The drawing under review shows one solid part. Ordinate dimensions are in mm from its lowest x, y, z. A direction names the side the tool comes from. Round coordinates to 2 decimals unless told otherwise and drop trailing zeros. Order: outer loops, then holes, each group sorted by start corner. A loop starts at its lowest first (then second) coordinate and runs counter-clockwise, first axis right, second up.
1) Consider section C-C (z = 79). Give the boundary of the cut face in (x, y).
2) Machinability: for the marked faces 1 and 2, which of the approach directions +Z, -Z, +X, -X, +Y, -Y give a long, thin tool a straight path to every point of the face, cutting with its end or side? Answer none if there is none.
3) Consider section A-A (y = 32). Give the boundary of the cut face in (x, z), then the cut area to 3 significant figures.
4) Consider section B-B (z = 54). Give the boundary of the cut face in (x, y).
5) Consider section D-D (x = 21.5). Give the boundary of the cut face in (y, z).
6) Clearance check with flat-ended pins moving along their axes: P1, Ø4, axis at x = 11.5, z = 18, coming from the +Y side; P2, Ø5, axis at y = 23, z = 21, coming from the +X side; P3, Ø12, axis at x = 11, y = 11, coming from the +Z side. State where each tip first meets the part, or that it passes through.
7) To check wall thickness, follow L1, parallel to Y at x = 11, z = 67. State the ranges of the line that lie inside material, in increasing order.
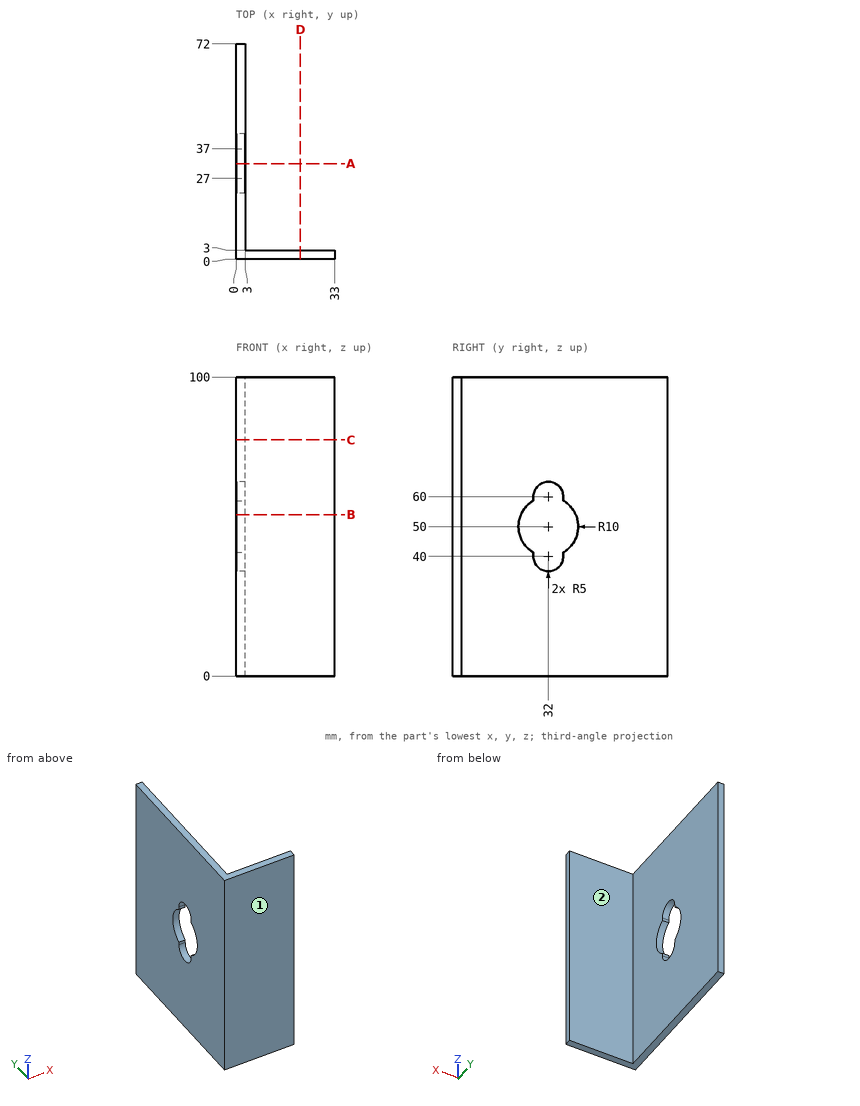
Answer below:
1. outline: (0, 0) - (33, 0) - (33, 3) - (3, 3) - (3, 72) - (0, 72) - close
2. face 1: +Z, -Z, +X, -X, -Y
2. face 2: +Z, -Z, +X, +Y
3. outline: (0, 0) - (3, 0) - (3, 35) - (0, 35) - close; (0, 65) - (3, 65) - (3, 100) - (0, 100) - close
3. area: 210 mm2
4. outline: (0, 0) - (33, 0) - (33, 3) - (3, 3) - (3, 22.83) - (0, 22.83) - close; (0, 41.17) - (3, 41.17) - (3, 72) - (0, 72) - close
5. outline: (0, 0) - (3, 0) - (3, 100) - (0, 100) - close
6. P1: stops at y = 3
6. P2: stops at x = 3
6. P3: passes through
7. L1: y = 0 to 3
